Design review of the part built by this model. Coordinates are the model's own, in mm. A direction names the side the tool comes from. Give positions to 0.01 mm unless a question says otherwise; leave off trailing zeros. Write each loop counter-clockwise with the first axis right and the second up, starting at its lowest first coordinate (ties: lowest second). Pieces come first, ordered by that corner, then holes. Notation, with made-up numbers: (0, -27) -> (52, -27) arc R19 cw to (52, -6) -> close; hole circle Ø8 at (4, 38.25). An arc over 180 degrees is marked (long way). Put each result on its own line as item: value. Start each with the question number.
from build123d import *

# Parameters (mm, degrees)
SKETCH1_W           = 33
SKETCH1_H           = 39
BOSS_EXTRUDE1_DEPTH = 13
SKETCH2_W           = 29.5
SKETCH2_H           = 35.5
CUT_EXTRUDE1_DEPTH  = 11
SKETCH3_R           = 1.85
SKETCH3_R_2         = 2
CUT_EXTRUDE2_DEPTH  = 57
SKETCH4_W           = 33
SKETCH4_H           = 39
BOSS_EXTRUDE2_DEPTH = 51.749999878


with BuildPart() as part:
    # Sketch1 → Boss-Extrude1 (new body)
    with BuildSketch(Plane(origin=(0, 0, 0), x_dir=(1, 0, 0), z_dir=(0, 1, 0))):
        with Locations((-45.059131656, -24.092112369)):
            Rectangle(SKETCH1_W, SKETCH1_H)
    extrude(amount=BOSS_EXTRUDE1_DEPTH)

    # Sketch2 → Cut-Extrude1 (cut)
    with BuildSketch(Plane(origin=(0, 13, 0), x_dir=(1, 0, 0), z_dir=(0, 1, 0))):
        with Locations((-45.059131656, -24.092112369)):
            Rectangle(SKETCH2_W, SKETCH2_H)
    extrude(amount=-CUT_EXTRUDE1_DEPTH, mode=Mode.SUBTRACT)

    # Sketch3 → Cut-Extrude2 (cut)
    with BuildSketch(Plane.XY.offset(43.592112369)):
        with Locations((-34.059131656, 5.4)):
            Circle(SKETCH3_R)
        with Locations((-56.059131656, 5.4)):
            Circle(SKETCH3_R_2)
    extrude(amount=-CUT_EXTRUDE2_DEPTH, mode=Mode.SUBTRACT)

    # Sketch4 → Boss-Extrude2 (add)
    with BuildSketch(Plane.XZ):
        with Locations((-45.059131656, 24.092112369)):
            Rectangle(SKETCH4_W, SKETCH4_H)
    extrude(amount=BOSS_EXTRUDE2_DEPTH)

    # Mirror7: part across plane


with BuildPart() as part_1:
    add(part.part)
    add(part.part.mirror(Plane.ZX.offset(-51.749999878)))


solid = part_1.part
Q1. Take a section at C-C on z = 23. Give the boundary of the cut face in (x, y), then the cut area to 3 significant figures.
Q2. To check wall thickness, follow probe 1 along Y at (x, z) = (-34, 42.5); probe 2 along X at (y, z) = (5, 43); probe 3 along Y at (x, z) = (-34.5, 40). State the ranges of each line that lie inside material, in increasing order. Write a range as from..to.
Q3. Mouldability with a two-part tool opening along Z and no side actions: class faces 1 (the face through (-45, -53, 43.592)), 2 (the face through (-56.493, -106.948, 42.729)), 3 (the face through (-30.309, -111, 24)) as +Z half, -Z half, draft (parallel to the pull), parting line (faces both ways), or undercut.
Q4. Machinability: for faces 4 (the face through (-45, -105.5, 24)), 5 (the face through (-30.309, 8, 24)), 6 (the face through (-28.559, -53, 24)), which of the approach directions +Z, -Z, +X, -X, +Y, -Y give a long, thin tool a straight path to every point of the face, cutting with its end or side? Answer none if there is none.
Q5. Take a section at A-A on y = 5.4. Give the boundary of the cut face in (x, z), then the cut area to 3 significant figures.
Q6. Take a section at B-B on x = -42.5. Give the boundary of the cut face in (y, z).
Q7. For pin 1 (2 mm diameter, centred on x = -37, z = 31, fed in from -Y); pin 2 (6 mm diameter, centred on x = -34.06, y = -108.9, fed in from -Z); pin 3 (12 mm diameter, centred on x = -48, z = 34, fed in from +Y), all flat-tipped, find the tip position at first contact; note any pin that passes through.
Result:
1. outline: (-61.56, -116.5) -> (-59.81, -116.5) -> (-59.81, -105.5) -> (-30.31, -105.5) -> (-30.31, -116.5) -> (-28.56, -116.5) -> (-28.56, 13) -> (-30.31, 13) -> (-30.31, 2) -> (-59.81, 2) -> (-59.81, 13) -> (-61.56, 13) -> close
1. area: 3,620 mm^2
2. probe 1: y = -116.5..-110.75, -107.05..3.55, 7.25..13
2. probe 2: x = -61.56..-58.02, -54.1..-35.87, -32.25..-28.56
2. probe 3: y = -105.5..2
3. face 1: +Z half
3. face 2: draft
3. face 3: undercut
4. face 4: -Y
4. face 5: +Y
4. face 6: +Z, -Z, +X, +Y, -Y
5. outline: (-61.56, 4.59) -> (-58.06, 4.59) -> (-58.06, 6.34) -> (-59.81, 6.34) -> (-59.81, 41.84) -> (-58.06, 41.84) -> (-58.06, 43.59) -> (-61.56, 43.59) -> close; (-54.06, 4.59) -> (-35.91, 4.59) -> (-35.91, 6.34) -> (-54.06, 6.34) -> close; (-54.06, 41.84) -> (-35.91, 41.84) -> (-35.91, 43.59) -> (-54.06, 43.59) -> close; (-32.21, 4.59) -> (-28.56, 4.59) -> (-28.56, 43.59) -> (-32.21, 43.59) -> (-32.21, 41.84) -> (-30.31, 41.84) -> (-30.31, 6.34) -> (-32.21, 6.34) -> close
5. area: 213 mm^2
6. outline: (-116.5, 4.59) -> (13, 4.59) -> (13, 6.34) -> (2, 6.34) -> (2, 41.84) -> (13, 41.84) -> (13, 43.59) -> (-116.5, 43.59) -> (-116.5, 41.84) -> (-105.5, 41.84) -> (-105.5, 6.34) -> (-116.5, 6.34) -> close
7. pin 1: stops at y = -105.5
7. pin 2: stops at z = 4.59
7. pin 3: stops at y = 2
